from build123d import *

# Parameters (mm, degrees)
F1_DEPTH      = 80
F3_DEPTH      = 37.501
F3_DEPTH_BACK = 52.501
F4_W          = 15
F4_H          = 6
F5_DEPTH      = 5
F7_DEPTH      = 30
F7_DEPTH_BACK = 15


with BuildPart() as f1:
    # F0 (on Top) → F1 (new body)
    with BuildSketch(Plane.XY):
        Polygon((-38.7530495245, 32.8086880944), (-45, 25), (-7.5, -5), (-7.5, -45), (7.5, -45), (7.5, -5), (45, 25), (38.7530495245, 32.8086880944), (0, 12.8086880944), align=None)
    extrude(amount=F1_DEPTH)

    # F2 (on face) → F3 (cut, two sides)
    with BuildSketch(Plane(origin=(-7.5, 0, 0), x_dir=(0, -1, 0), z_dir=(-1, 0, 0))) as f3_sk:
        Polygon((45, 23.9833969432), (45, 80), (-35, 80), align=None)
    extrude(amount=F3_DEPTH, mode=Mode.SUBTRACT)
    extrude(f3_sk.sketch, amount=-F3_DEPTH_BACK, mode=Mode.SUBTRACT)

    # F4 (on face) → F5 (join)
    with BuildSketch(Plane(origin=(0, -26.0730573396, 37.2361848693), x_dir=(1, 0, 0), z_dir=(0, -0.5735764364, 0.8191520443))):
        Polygon((-42.207332973, 66.6102117473), (-45, 62.3486905706), (-37.8457929426, 55.3617512278), (-34.3523232712, 58.9388547565), align=None)
        Polygon((37.8457929426, 55.3617512278), (45, 62.3486905706), (42.207332973, 66.6102117473), (34.3523232712, 58.9388547565), align=None)
        with Locations((0, -20.1055306427)):
            Rectangle(F4_W, F4_H)
    extrude(amount=F5_DEPTH)

    # F6 (on face) → F7 (cut, two sides)
    with BuildSketch(Plane(origin=(-7.5, 0, 0), x_dir=(0, -1, 0), z_dir=(-1, 0, 0))) as f7_sk:
        Polygon((-25.014819764, 45), (14.985180236, 45), (-25.014819764, 73.0083015284), align=None)
    extrude(amount=-F7_DEPTH, mode=Mode.SUBTRACT)
    extrude(f7_sk.sketch, amount=F7_DEPTH_BACK, mode=Mode.SUBTRACT)


solid = f1.part
Geometry: final body of the model. Coordinates: model frame, mm. A direction names the side the tool comes from. Round coordinates to 2 decimals unless told otherwise and drop trailing zeros. Write each loop counter-clockwise with the first axis right and the second up, starting at its lowest first coordinate (ties: lowest second). Pieces come first, ordered by that corner, then holes. Notation, with made-up numbers: M 45.25,7.25 L 92.25,7.25 A15 ccw 92.25,36.25 Z; hole C 22.5,51.5 d1. An arc over 180 degrees is marked long. Write item = value, one per line.
Item 1: Section query B-B on z = 18.5. Return loops of the section in (x, y).
Findings:
outline = M -45,25 L -7.5,-5 L -7.5,-45 L 7.5,-45 L 7.5,-5 L 45,25 L 38.75,32.81 L 0,12.81 L -38.75,32.81 Z
Item 2: Section query D-D on x = -5. Return loops of the section in (y, z).
Findings:
outline = M -47.87,28.08 L -45,23.98 L -45,0 L 15.39,0 L 15.39,45 L -14.99,45 L -40.09,27.42 L -42.95,31.52 Z
Item 3: Material intervals for line 1 along X through (y, z) = (-41, 18); line 2 along Z through (x, y) = (-15, 13.5); line 3 along Y through (x, z) = (-37, 75.5), sorted ascending. Write a range as [from, to].
Findings:
line_1 = [-7.5, 7.5]
line_2 = [0, 45]
line_3 = [19.86, 22.24], [28.57, 31.9]
Item 4: Section query C-C on y = 9.5. Return loops of the section in (x, z) (3 decimals), then the cut area to 3 significant figures.
Findings:
outline = M -25.625,0 L 25.625,0 L 25.625,62.145 L 22.5,62.145 L 22.5,45 L -22.5,45 L -22.5,62.145 L -25.625,62.145 Z
area = 2,410 mm^2
Item 5: Section query A-A on z = 67.5. Return loops of the section in (x, y).
Findings:
outline = M -45,25 L -35.19,17.15 L -22.5,17.15 L -22.5,24.42 L -38.75,32.81 Z; M 22.5,17.15 L 35.19,17.15 L 45,25 L 38.75,32.81 L 22.5,24.42 Z
Item 6: Pull-direction query (X, two-part tool) for faces 4 (the face through (0, -45, 12)), 5 (the face through (22.5, 16, 56)), 6 (the face through (-41.8, 29, 38.7)), 7 (the face through (-23.41, 24.89, 29.97)); classes: pulls with the +X half, pulls with the -X half, needs draft (parallel to the pull), parting line crosses it, or undercut.
Findings:
face_4 = needs draft
face_5 = undercut
face_6 = pulls with the -X half
face_7 = undercut
Item 7: Access query for faces 1 (the face through (-7.5, -21, 17)), 2 (the face through (0.105, -27.359, 36.335)), 3 (the face through (7.5, -22, 17)). Directions: +Z, -Z, +X, -X, +Y, -Y. A direction counts if a zero-diameter tool reaches every point of the face in a straight line with its end or side. Return the directions, or none.
Findings:
face_1 = +Z, -Z, -X, -Y
face_2 = +Z, +X, -X
face_3 = +Z, -Z, +X, -Y
Item 8: Pin query (flat end, axial travel): P1, Ø21.5, axis at y = -31.5, z = 27, coming from the -X side; P2, Ø6, axis at x = 15.5, y = 1, coming from the +Z side; P3, Ø19, axis at y = 11.5, z = 64.5, coming from the +X side. Return the tip coordinate at first contact, or that it passes through.
Findings:
P1 = -7.5
P2 = 45
P3 = 40
